Source: CAD feature listing. Evaluate the final solid. Frame: model axes, mm. Face numbers are marked on the shaded views. A direction names the side the tool comes from. Coordinates: 2 decimals unless noted, no trailing zeros. Write each loop counter-clockwise with the first axis right and the second up, starting at its lowest first coordinate (ties: lowest second). Pieces come first, ordered by that corner, then holes. Notation, with made-up numbers: (16, 55.25) -> (68, 55.25) arc R12 cw to (68, 65.25) -> close; hole circle Ø5 at (16, 49.25). An arc over 180 degrees is marked (long way). Write item = value, one per line.
from build123d import *

# Parameters (mm, degrees)
SKETCH1_W           = 40
SKETCH1_H           = 40
SKETCH1_R           = 5
SKETCH1_R_2         = 1.65
SKETCH1_R_3         = 1.5
BOSS_EXTRUDE1_DEPTH = 6
SKETCH2_W           = 6
SKETCH2_H           = 25.5
BOSS_EXTRUDE2_DEPTH = 40
SKETCH3_R           = 3.5
CUT_EXTRUDE1_DEPTH  = 3
FILLET1_R           = 10


with BuildPart() as part:
    # Sketch1 → Boss-Extrude1 (new body)
    with BuildSketch(Plane.XY):
        with Locations((20, 20)):
            Rectangle(SKETCH1_W, SKETCH1_H)
        with Locations((20, 20)):
            Circle(SKETCH1_R, mode=Mode.SUBTRACT)
        with Locations((12, 28)):
            Circle(SKETCH1_R_2, mode=Mode.SUBTRACT)
        with Locations((20, 29.192388155)):
            Circle(SKETCH1_R_3, mode=Mode.SUBTRACT)
        with Locations((29.192388155, 20)):
            Circle(SKETCH1_R_3, mode=Mode.SUBTRACT)
        with Locations((20, 10.807611845)):
            Circle(SKETCH1_R_3, mode=Mode.SUBTRACT)
        with Locations((10.807611845, 20)):
            Circle(SKETCH1_R_3, mode=Mode.SUBTRACT)
        with Locations((28, 28)):
            Circle(SKETCH1_R_2, mode=Mode.SUBTRACT)
        with Locations((12, 12)):
            Circle(SKETCH1_R_2, mode=Mode.SUBTRACT)
        with Locations((28, 12)):
            Circle(SKETCH1_R_2, mode=Mode.SUBTRACT)
    extrude(amount=BOSS_EXTRUDE1_DEPTH)

    # Sketch2 → Boss-Extrude2 (add)
    with BuildSketch(Plane(origin=(40, 0, 0), x_dir=(0, 0, -1), z_dir=(1, 0, 0))):
        Polygon((44, 0), (-6, 0), (-6, -4), (0, -4), (44, -4), align=None)
        with Locations((-3, -16.75)):
            Rectangle(SKETCH2_W, SKETCH2_H)
        Polygon((0, -29.5), (-6, -29.5), (-6, -33.5), (44, -33.5), (44, -29.5), align=None)
    extrude(amount=-BOSS_EXTRUDE2_DEPTH)

    # Sketch3 → Cut-Extrude1 (cut)
    with BuildSketch(Plane(origin=(0, 0, 0), x_dir=(-1, 0, 0), z_dir=(0, 0, -1))):
        with Locations((-20, 29.192388155)):
            Circle(SKETCH3_R)
        with Locations((-20, 10.807611845)):
            Circle(SKETCH3_R)
        with Locations((-29.192388155, 20)):
            Circle(SKETCH3_R)
        with Locations((-10.807611845, 20)):
            Circle(SKETCH3_R)
    extrude(amount=-CUT_EXTRUDE1_DEPTH, mode=Mode.SUBTRACT)

    # Fillet1
    fillet1_edges = [part.edges().sort_by_distance(p)[0] for p in [
        (40, -2, -44),
        (0, -31.5, -44),
        (0, -2, -44),
        (40, -31.5, -44),
        (0, 40, 3),
        (40, 40, 3),
    ]]
    fillet(fillet1_edges, radius=FILLET1_R)


solid = part.part
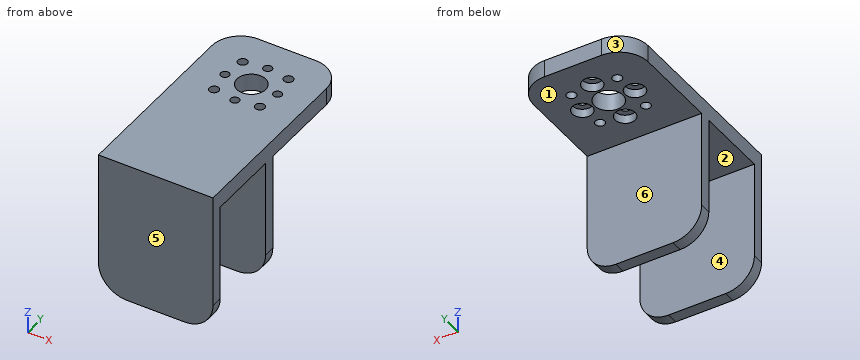
1) First-contact query: pin 1 Ø13 at (x, y) = (26, -21.5) entering from -Z; pin 2 Ø3.5 at (x, y) = (10, 21.5) entering from -Z; pin 3 Ø6 at (x, y) = (6.5, -3.5) entering from -Z; pin 4 Ø6.5 at (x, y) = (20, 10.81) entering from +Z. Flat tips, straight axial feed; report the tip coordinate or a pass-through.
Answer block:
pin_1 = 0
pin_2 = 3
pin_3 = -43.99
pin_4 = 6
2) Material intervals for probe 1 along Y at (x, z) = (29, -5); probe 2 along Y at (x, z) = (20, 4); probe 3 along Z at (x, y) = (25, 15), sorted ascending. Write a range as [from, to].
Answer block:
probe_1 = [-33.5, -29.5], [-4, 0]
probe_2 = [-33.5, 9.31], [12.31, 15], [25, 27.69], [30.69, 40]
probe_3 = [0, 6]
3) Pull-direction query (Y, two-part tool) for the marked faces 1, 2 and 3; classes: +Y half, -Y half, draft (parallel to the pull), parting line (faces both ways), or undercut.
Answer block:
face_1 = draft
face_2 = undercut
face_3 = +Y half
4) Cut plane B-B, the plane x = 20. Give the number of separate pieces and of enclosed holes in the cut face, and give its area (3 significant figures).
Answer block:
separate_pieces = 4
enclosed_holes = 0
area = 673 mm2
5) Cut plane D-D, the plane x = 4. Output: boundary loops of the cut face in (y, z).
Answer block:
outline = (-33.5, -42) -> (-29.5, -42) -> (-29.5, 0) -> (-4, 0) -> (-4, -42) -> (0, -42) -> (0, 0) -> (38, 0) -> (38, 6) -> (-33.5, 6) -> close
6) Reachability of the marked faces 4, 5 and 6 from +Z, -Z, +X, -X, +Y, -Y: full face, straight path, thin tool, end or side. Return the list, or none.
Answer block:
face_4 = -Z, +X, -X
face_5 = +Z, -Z, +X, -X, -Y
face_6 = -Z, +X, -X, +Y
7) Cut plane A-A, the plane y = 20. Output: boundary loops of the cut face in (x, z), and give its area (3 significant figures).
Answer block:
outline = (0, 0) -> (7.31, 0) -> (7.31, 3) -> (9.31, 3) -> (9.31, 6) -> (0, 6) -> close; (12.31, 3) -> (14.31, 3) -> (14.31, 0) -> (15, 0) -> (15, 6) -> (12.31, 6) -> close; (25, 0) -> (25.69, 0) -> (25.69, 3) -> (27.69, 3) -> (27.69, 6) -> (25, 6) -> close; (30.69, 3) -> (32.69, 3) -> (32.69, 0) -> (40, 0) -> (40, 6) -> (30.69, 6) -> close
area = 120 mm2
8) Cut plane C-C, the plane z = -37.5. Output: boundary loops of the cut face in (x, y).
Answer block:
outline = (0.63, -33.5) -> (39.37, -33.5) -> (39.37, -29.5) -> (0.63, -29.5) -> close; (0.63, -4) -> (39.37, -4) -> (39.37, 0) -> (0.63, 0) -> close
